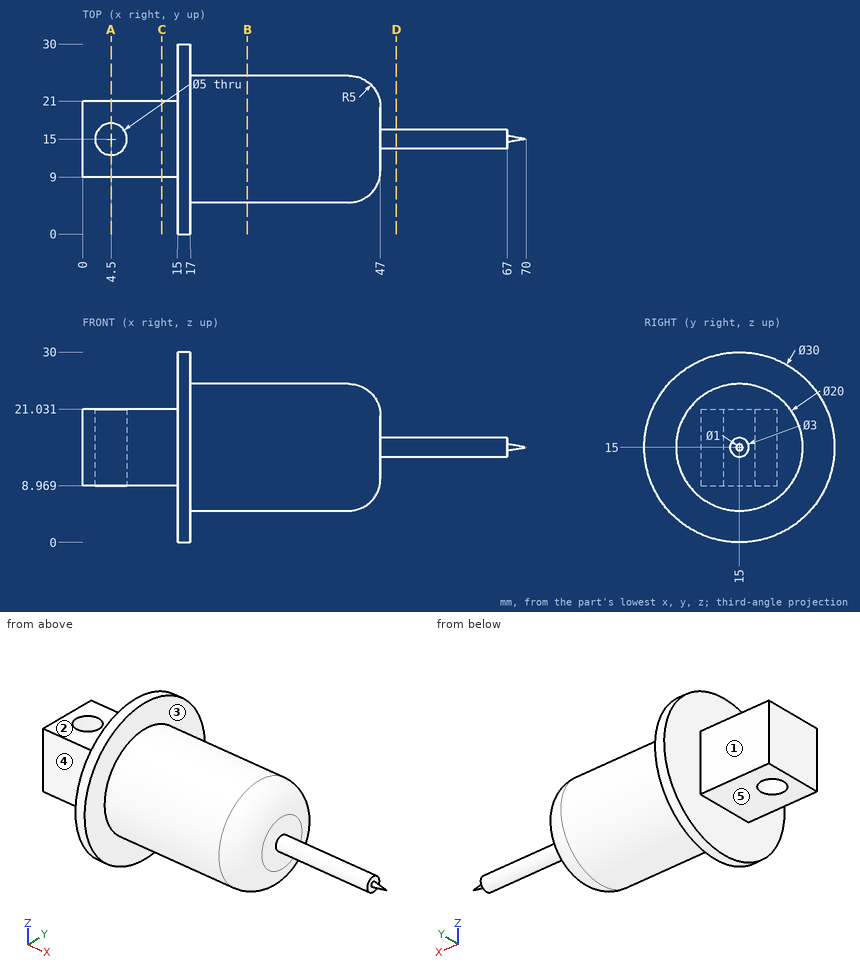
For this review, use the dimensioned drawing (mm, ordinates from the lowest corner) and the shaded views. A direction names the side the tool comes from. Round coordinates to 2 decimals unless told otherwise and drop trailing zeros. Write each loop counter-clockwise with the first axis right and the second up, starting at its lowest first coordinate (ties: lowest second). Pieces come first, ordered by that corner, then holes. Notation, with made-up numbers: (22.25, 72) -> (51.25, 72) arc R21 cw to (51.25, 88) -> close; hole circle Ø11 at (-20, 9). An arc over 180 degrees is marked (long way). Use one line per item in the form item = value.
Q1. Consider section B-B (x = 26). State the section outline as (y, z) points, then the cut area to 3 significant figures.
Resolved:
outline = circle Ø20 at (15, 15)
area = 314 mm²
Q2. Machinability: for the marked faces 1, 2, 3, 4 and 5, which of the approach directions +Z, -Z, +X, -X, +Y, -Y give a long, thin tool a straight path to every point of the face, cutting with its end or side? Answer none if there is none.
Resolved:
face_1 = +Z, -Z, -X, +Y
face_2 = +Z, -X, +Y, -Y
face_3 = +X
face_4 = +Z, -Z, -X, -Y
face_5 = -Z, -X, +Y, -Y
Q3. To check wall thickness, follow probe 1 along Y at (x, z) = (4.5, 13.5); probe 2 along Z at (x, y) = (23.5, 14.5); probe 3 along X at (y, z) = (4.5, 11.75). State the ranges of each line that lie inside material, in increasing order. Write a range as from..to.
Resolved:
probe_1 = 9..12.5, 17.5..21
probe_2 = 5.01..24.99
probe_3 = 15..17
Q4. Consider section D-D (x = 49.5). State the section outline as (y, z) points.
Resolved:
outline = circle Ø3 at (15, 15)
Q5. Consider section C-C (x = 12.5). State the section outline as (y, z) points, then the cut area to 3 significant figures.
Resolved:
outline = (9, 8.97) -> (21, 8.97) -> (21, 21.03) -> (9, 21.03) -> close
area = 145 mm²
Q6. Clearance check with flat-ended pins moving along their axes: pin 1 Ø6 at (x, y) = (10.5, 15) entering from +Z; pin 2 Ø3 at (x, y) = (4.5, 15) entering from +Z; pin 3 Ø3.5 at (x, z) = (5.5, 12) entering from +Y; pin 4 Ø2 at (x, y) = (33.5, 14) entering from -Z. State where each tip first meets the part, or that it passes through.
Resolved:
pin_1 = 21.03
pin_2 = through
pin_3 = 21
pin_4 = 5
Q7. Consider section A-A (x = 4.5). State the section outline as (y, z) points.
Resolved:
outline = (9, 8.97) -> (12.5, 8.97) -> (12.5, 21.03) -> (9, 21.03) -> close; (17.5, 8.97) -> (21, 8.97) -> (21, 21.03) -> (17.5, 21.03) -> close
